Source: CAD feature listing. Evaluate the final solid. Frame: model axes, mm. A direction names the side the tool comes from. Give positions to 0.01 mm unless a question says otherwise; leave off trailing zeros. Write each loop counter-clockwise with the first axis right and the second up, starting at its lowest first coordinate (ties: lowest second). Pieces come first, ordered by that corner, then holes. Notation, with made-up numbers: (2.5, 64) -> (56.5, 64) arc R16 cw to (56.5, 91) -> close; hole circle Ø7 at (34.5, 37.5). An arc over 180 degrees is marked (long way). Answer as a JSON object with one key per item and string values. Group by question number.
Item 1: Access query for faces 4 (the face through (-0.067, 5.324, -6.944)), 5 (the face through (0.09, -0.54, -2.44)). Directions: +Z, -Z, +X, -X, +Y, -Y. A direction counts if a zero-diameter tool reaches every point of the face in a straight line with its end or side. Return the directions, or none.
Item 2: Section query C-C on x = 0.5. Return the cut outline in (y, z).
Item 3: Pull-direction query (X, two-part tool) for faces 1 (the face through (-4.75, 9, 1)), 2 (the face through (-5.56, 10.74, -2.38)), 3 (the face through (-6.35, -3, 0)); classes: pulls with the +X half, pulls with the -X half, needs draft (parallel to the pull), parting line crosses it, or undercut.
Item 4: Ray query, probe 1 along X at (y, z) = (-10, 3.75); probe 2 along Z at (x, y) = (-1, 0); probe 3 along Z at (x, y) = (-1.25, -0.5). Return the intervals inside material, ascending. Write a range as from..to.
Item 5: Section query A-A on y = 0. Return the cut outline in (x, z), plus the area to 3 significant figures.
Item 6: Section query D-D on y = 6.25. Return the cut outline in (x, z).
Item 7: First-contact query: pin 1 Ø1 at (x, z) = (-5, -5) entering from -Y; pin 2 Ø4 at (x, y) = (4, 7) entering from -Z; pin 3 Ø6 at (x, y) = (0.5, 5.5) entering from -Z. Flat tips, straight axial feed; report the tip coordinate or a pass-through.
from build123d import *

# Parameters (mm, degrees)
F2_R     = 2.5
F3_DEPTH = 12.701


with BuildPart() as f1:
    # F0 (on Front) → F1 (revolve)
    with BuildSketch(Plane.XZ):
        Polygon((-6.35, 11), (-6.35, 0), (6.35, 0), (6.35, 11), (4.75, 11), (4.75, 8.75), (-4.75, 8.75), (-4.75, 11), align=None)
    revolve(axis=Axis((-12.864703, 0, 0), (1, 0, 0)))

    # F2 (on face) → F3 (cut, through all)
    with BuildSketch(Plane.YZ.offset(6.35)):
        Circle(F2_R)
    extrude(amount=-F3_DEPTH, mode=Mode.SUBTRACT)


solid = f1.part
Worked answers:
{
 "1": {"face 4": "none", "face 5": "+X, -X"},
 "2": {"outline": "circle Ø17.5 at (0, 0); hole circle Ø5 at (0, 0)"},
 "3": {"face 1": "undercut", "face 2": "needs draft", "face 3": "pulls with the -X half"},
 "4": {"probe 1": "-6.35..-4.75, 4.75..6.35", "probe 2": "-8.75..-2.5, 2.5..8.75", "probe 3": "-8.74..-2.45, 2.45..8.74"},
 "5": {"outline": "(-6.35, -11) -> (-4.75, -11) -> (-4.75, -8.75) -> (4.75, -8.75) -> (4.75, -11) -> (6.35, -11) -> (6.35, -2.5) -> (-6.35, -2.5) -> close; (-6.35, 2.5) -> (6.35, 2.5) -> (6.35, 11) -> (4.75, 11) -> (4.75, 8.75) -> (-4.75, 8.75) -> (-4.75, 11) -> (-6.35, 11) -> close", "area": "173 mm^2"},
 "6": {"outline": "(-6.35, -9.05) -> (-4.75, -9.05) -> (-4.75, -6.12) -> (4.75, -6.12) -> (4.75, -9.05) -> (6.35, -9.05) -> (6.35, 9.05) -> (4.75, 9.05) -> (4.75, 6.12) -> (-4.75, 6.12) -> (-4.75, 9.05) -> (-6.35, 9.05) -> close"},
 "7": {"pin 1": "y = -10.04", "pin 2": "z = -9.72", "pin 3": "z = -8.39"}
}
